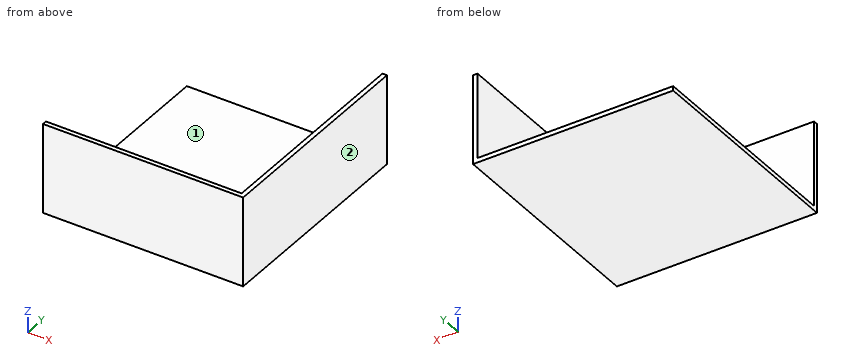
from build123d import *

# Parameters (mm, degrees)
F0_W     = 277.368
F0_H     = 303.784
F1_DEPTH = 6.35
F2_W     = 277.368
F2_H     = 127
F2_H_2   = 120.65
F3_DEPTH = 6.35
F4_W     = 310.134
F4_H     = 127
F5_DEPTH = 6.35


with BuildPart() as f1:
    # F0 (on Top) → F1 (new body)
    with BuildSketch(Plane.XY):
        with Locations((138.684, 151.892)):
            Rectangle(F0_W, F0_H)
    extrude(amount=F1_DEPTH)

    # F2 (on face) → F3 (join)
    with BuildSketch(Plane.XZ):
        with Locations((138.684, 63.5)):
            Rectangle(F2_W, F2_H)
        with Locations((138.684, 66.675)):
            Rectangle(F2_W, F2_H_2)
    extrude(amount=F3_DEPTH)

    # F4 (on face) → F5 (join)
    with BuildSketch(Plane.YZ.offset(277.368)):
        with Locations((148.717, 63.5)):
            Rectangle(F4_W, F4_H)
        Polygon((-6.35, 127), (-6.35, 0), (303.784, 0), (303.784, 6.35), (0, 6.35), (0, 127), align=None)
    extrude(amount=F5_DEPTH)


solid = f1.part
Can you work these out from the model? Positions are in its coordinate system, mm. Face numbers are marked on the shaded views. A direction names the side the tool comes from. Give positions to 0.01 mm unless a question says otherwise; leave off trailing zeros. Order: outer loops, then holes, each group sorted by start corner. A loop starts at its lowest first (then second) coordinate and runs counter-clockwise, first axis right, second up. Notation, with made-up numbers: M 80,3.5 L 105,3.5 A33 cw 105,35.5 Z; hole C 40.25,77 d6. An arc over 180 degrees is marked long. One line per item, written item: value.
Item 1: If we section it at B-B on z = 60: Write out the boundary of the cut face in (x, y).
Verdict:
outline: M 0,-6.35 L 283.72,-6.35 L 283.72,303.78 L 277.37,303.78 L 277.37,0 L 0,0 Z
Item 2: For the marked faces 1 and 2, which set-ups out of +Z, -Z, +X, -X, +Y, -Y let a thin tool reach every point of the face, with its end or its side?
Verdict:
face 1: +Z, -X, +Y
face 2: +Z, -Z, +X, +Y, -Y
Item 3: For pin 1 (1 mm diameter, centred on x = 230, y = 240.5, fed in from +Z); pin 2 (1.5 mm diameter, centred on y = 213.5, z = 26.5, fed in from -X); pin 3 (6 mm diameter, centred on x = 198, z = 15.5, fed in from +Y), each with a flat end and sliding along its axis, tell me the tip position at first contact or that it passes through.
Verdict:
pin 1: z = 6.35
pin 2: x = 277.37
pin 3: y = 0
Item 4: If we section it at A-A on x = 264: Write out the boundary of the cut face in (y, z).
Verdict:
outline: M -6.35,0 L 303.78,0 L 303.78,6.35 L 0,6.35 L 0,127 L -6.35,127 Z
Item 5: Please list where these lines run through material, in increasing order: line 1 (X direction, y = 195, z = 66.5); line 2 (Z direction, x = 40, y = 214); line 3 (Y direction, x = 24.5, z = 79.5).
Verdict:
line 1: 277.37 to 283.72
line 2: 0 to 6.35
line 3: -6.35 to 0
